Build history of the part. All positions in model axes, mm. A direction names the side the tool comes from. Round coordinates to 2 decimals unless told otherwise and drop trailing zeros. Write each loop counter-clockwise with the first axis right and the second up, starting at its lowest first coordinate (ties: lowest second). Pieces come first, ordered by that corner, then holes. Notation, with made-up numbers: (54.25, -16.5) - (70.25, -16.5) arc R15 ccw to (70.25, -8.5) - close; hole circle Ø6 at (28.25, -29.75). An arc over 180 degrees is marked (long way). Write each question's results on one line, items separated by ' | '.
from build123d import *

# Parameters (mm, degrees)
SKETCH_R           = 10
SKETCH_W           = 14.142136
SKETCH_H           = 14.142136
PAD_DEPTH          = 1.85
SKETCH001_W        = 40
SKETCH001_H        = 320
POCKET_DEPTH       = 100
POCKET_DEPTH_BACK  = 100
POCKET002_START    = 0.85
SKETCH003_R        = 4.25
POCKET002_DEPTH    = 99.15
SKETCH004_R        = 5
PAD001_DEPTH       = 0.5
SKETCH002_R        = 1.25
POCKET001_DEPTH    = 50
POLARPATTERN_COUNT = 4


with BuildPart() as part:
    # Sketch → Pad (new body)
    with BuildSketch(Plane.XY):
        with Locations((0, 40)):
            Circle(SKETCH_R)
        Polygon((0, 90), (-8.660254, 75), (8.660254, 75), align=None)
        with Locations((0, 120)):
            Rectangle(SKETCH_W, SKETCH_H)
        Polygon((0, 10), (-9.510565, 3.09017), (-5.877853, -8.09017), (5.877853, -8.09017), (9.510565, 3.09017), align=None)
        Polygon((-8.660254, 205), (-8.660254, 195), (0, 190), (8.660254, 195), (8.660254, 205), (0, 210), align=None)
    extrude(amount=PAD_DEPTH)

    # Sketch001 → Pocket (cut, two sides)
    with BuildSketch(Plane.XY) as pocket_sk:
        with Locations((0, 180.01)):
            Rectangle(SKETCH001_W, SKETCH001_H)
    extrude(amount=POCKET_DEPTH, mode=Mode.SUBTRACT)
    extrude(pocket_sk.sketch, amount=-POCKET_DEPTH_BACK, mode=Mode.SUBTRACT)

    # Sketch003 → Pocket002 (cut)
    with BuildSketch(Plane.XY.offset(POCKET002_START)):
        Circle(SKETCH003_R)
    extrude(amount=POCKET002_DEPTH, mode=Mode.SUBTRACT)

    # Sketch004 → Pad001 (join)
    with BuildSketch(Plane.XY):
        Circle(SKETCH004_R)
    extrude(amount=-PAD001_DEPTH)

    # Sketch002 → Pocket001 (cut, symmetric)
    with BuildSketch(Plane.XY):
        with Locations((-4.25, 0)):
            Circle(SKETCH002_R)
    pocket001 = extrude(amount=POCKET001_DEPTH, both=True, mode=Mode.SUBTRACT)

    # PolarPattern: Pocket001 ×4 about axis
    polarpattern_axis = Axis((0, 0, 0), (0, 0, 1))
    for i in range(1, POLARPATTERN_COUNT):
        add(pocket001.rotate(polarpattern_axis, i * 360 / POLARPATTERN_COUNT), mode=Mode.SUBTRACT)


solid = part.part
(1) Slice it at B-B, the plane y = 0. Write the cut outline in (x, z).
Worked answers:
outline: (-8.51, 0) - (-5.5, 0) - (-5.5, 1.85) - (-8.51, 1.85) - close; (-3, -0.5) - (3, -0.5) - (3, 0.85) - (-3, 0.85) - close; (5.5, 0) - (8.51, 0) - (8.51, 1.85) - (5.5, 1.85) - close
(2) Two-plate mould, pull along X, no slides. Class faces 1 (the flat face through (7.67, -2.58, 0.91)), 2 (the cylindrical face through (-3.56, -3.51, -0.25)), 3 (the cylindrical face through (5.5, -0.05, 0.69)): released by +X, released by -X, zero draft, split by the parting line, or undercut.
Worked answers:
face 1: released by +X | face 2: released by -X | face 3: undercut
(3) Slice it at D-D, the plane y = -4.5. Write the cut outline in (x, z).
Worked answers:
outline: (-7.04, 0) - (-2.18, 0) - (-2.18, -0.5) - (-1.22, -0.5) - (-1.22, 1.85) - (-7.04, 1.85) - close; (1.22, -0.5) - (2.18, -0.5) - (2.18, 0) - (7.04, 0) - (7.04, 1.85) - (1.22, 1.85) - close
(4) Slice it at A-A, the plane z = 1.4. Write the cut outline in (x, y).
Worked answers:
outline: (-9.51, 3.09) - (-5.88, -8.09) - (5.88, -8.09) - (9.51, 3.09) - (0, 10) - close; hole (-4.07, -1.24) arc R4.25 ccw to (-1.24, -4.07) arc R1.25 ccw (long way) to (1.24, -4.07) arc R4.25 ccw to (4.07, -1.24) arc R1.25 ccw (long way) to (4.07, 1.24) arc R4.25 ccw to (1.24, 4.07) arc R1.25 ccw (long way) to (-1.24, 4.07) arc R4.25 ccw to (-4.07, 1.24) arc R1.25 ccw (long way) to start
(5) Flat gauge pins, fed straight in: pin 1 Ø2 at (x, y) = (0, -4.25) entering from -Z; pin 2 Ø3 at (x, y) = (6.5, 0) entering from -Z; pin 3 Ø1 at (y, z) = (4, 1) entering from +X; pin 4 Ø2.5 at (x, y) = (1.5, 0) entering from +Z. Where does each tip first touch, or does it go through?
Worked answers:
pin 1: passes through | pin 2: stops at z = 0 | pin 3: stops at x = 8.95 | pin 4: stops at z = 0.85
(6) Drill centre lines: probe 1 along X at (y, z) = (0, 0.15); probe 2 along Z at (x, y) = (6, -0.5); probe 3 along Y at (x, z) = (-4.5, 1.4). Where is each one in solid material? Low to high. Write a range as [from, to].
Worked answers:
probe 1: x = [-8.51, -5.5], [-3, 3], [5.5, 8.51] | probe 2: z = [0, 1.85] | probe 3: y = [-8.09, -1.22], [1.22, 6.73]
(7) Slice it at C-C, the plane z = 0.4. Write the cut outline in (x, y).
Worked answers:
outline: (-9.51, 3.09) - (-5.88, -8.09) - (5.88, -8.09) - (9.51, 3.09) - (0, 10) - close; hole circle Ø2.5 at (-4.25, 0); hole circle Ø2.5 at (0, -4.25); hole circle Ø2.5 at (0, 4.25); hole circle Ø2.5 at (4.25, 0)
(8) Tool access for faces 4 (the cylindrical face through (3.51, -3.56, -0.25)), 5 (the cylindrical face through (-3.51, 3.56, -0.25)), 6 (the flat face through (0, 0, 0.85)): list every direction of +Z, -Z, +X, -X, +Y, -Y with a clear straight run to the whole face (end or side of a thin tool).
Worked answers:
face 4: -Z, +X, -Y | face 5: -Z, -X, +Y | face 6: +Z
